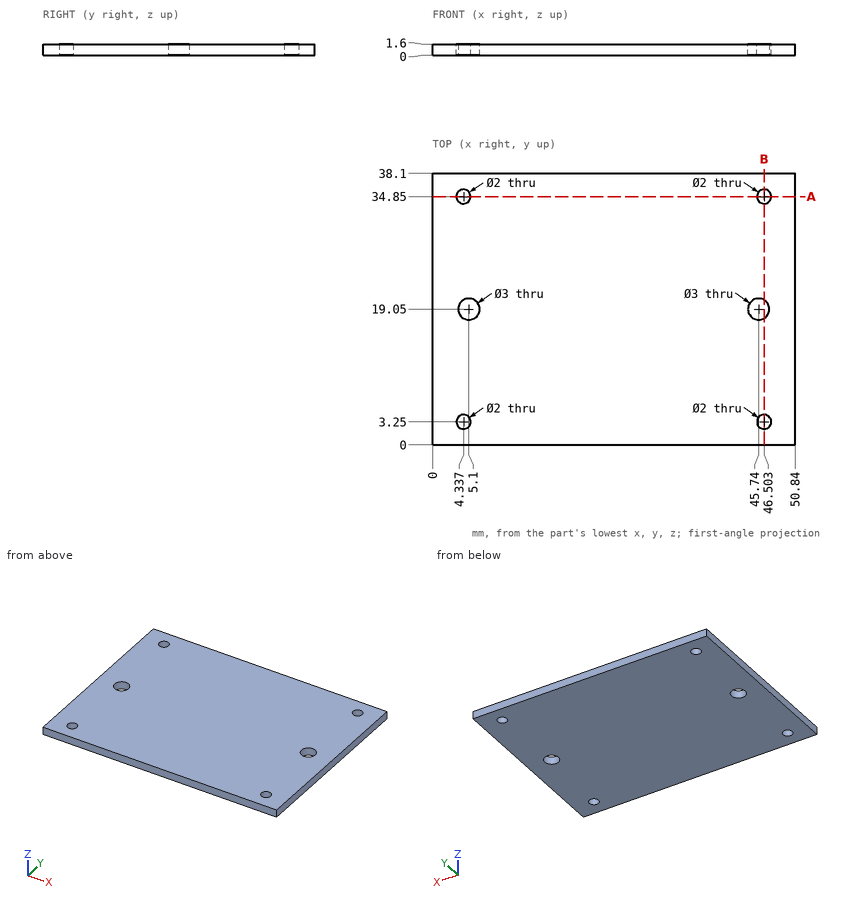
Could you check a few things on this drawing? It's one solid part, dimensions in mm from its lowest x, y, z. Give positions to 0.01 mm unless a question says otherwise; leave off trailing zeros. Order: outer loops, then holes, each group sorted by start corner. A loop starts at its lowest first (then second) coordinate and runs counter-clockwise, first axis right, second up. Notation, with made-up numbers: (2, -2.75) -> (9, -2.75) arc R12 ccw to (9, 8.25) -> close; hole circle Ø3 at (-26, 1). An arc over 180 degrees is marked (long way). Answer in a Markdown table with one row per item. Add a question column.
Item 1: Please list where these lines run through material, in increasing order: probe 1 along X at (y, z) = (35, 1.25) (1 decimal); probe 2 along X at (y, z) = (18, 1.1); probe 3 along Y at (x, z) = (4, 0.8).
Item 2: Imagine slicing it at A-A (y = 34.85). List the corners of the cut face in (x, z) for me.
Item 3: I'm going to push a flat-ended pin straight in: P1, Ø1.6, axis at x = 46.5, y = 34.85, coming from the -Z side. Where does the tip first touch, or does it pass through?
Item 4: Imagine slicing it at B-B (x = 46.5). List the corners of the cut face in (y, z) for me.
Result:
| question | item | result |
|---|---|---|
| 1 | probe 1 | 0 to 3.3, 5.3 to 45.5, 47.5 to 50.8 |
| 1 | probe 2 | 0 to 4.03, 6.17 to 44.67, 46.81 to 50.84 |
| 1 | probe 3 | 0 to 2.31, 4.19 to 18.03, 20.07 to 33.91, 35.79 to 38.1 |
| 2 | outline | (0, 0) -> (3.34, 0) -> (3.34, 1.6) -> (0, 1.6) -> close; (5.34, 0) -> (45.5, 0) -> (45.5, 1.6) -> (5.34, 1.6) -> close; (47.5, 0) -> (50.84, 0) -> (50.84, 1.6) -> (47.5, 1.6) -> close |
| 3 | P1 | through |
| 4 | outline | (0, 0) -> (2.25, 0) -> (2.25, 1.6) -> (0, 1.6) -> close; (4.25, 0) -> (17.76, 0) -> (17.76, 1.6) -> (4.25, 1.6) -> close; (20.34, 0) -> (33.85, 0) -> (33.85, 1.6) -> (20.34, 1.6) -> close; (35.85, 0) -> (38.1, 0) -> (38.1, 1.6) -> (35.85, 1.6) -> close |
